Here's the drawing with two shaded views (mm, measured from the low corner). I have some questions. Round coordinates to 2 decimals unless told otherwise and drop trailing zeros. Order: outer loops, then holes, each group sorted by start corner. A loop starts at its lowest first (then second) coordinate and runs counter-clockwise, first axis right, second up. Notation, with made-up numbers: (-22, -35.5) -> (1, -35.5) arc R7 cw to (1, -22.5) -> close; hole circle Ø1 at (-24.5, 45). An arc over 180 degrees is marked (long way). Answer in a Markdown table with one row per item.
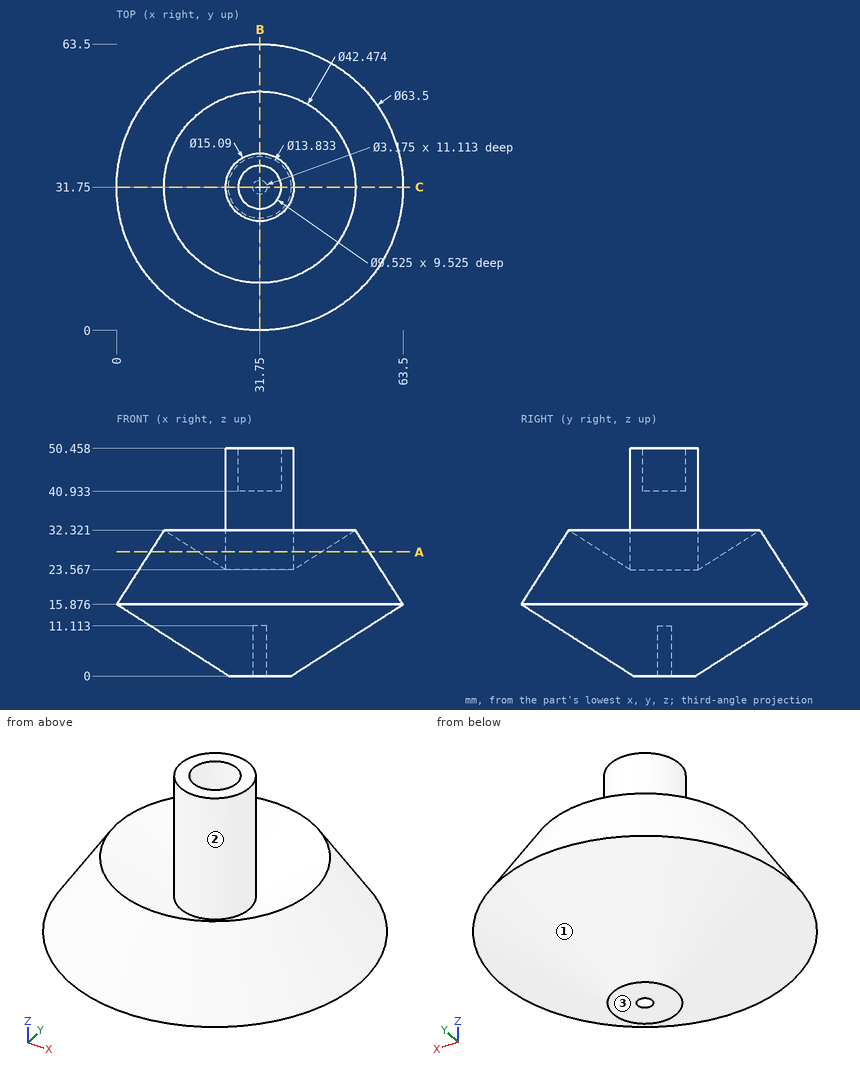
1. We'd pull the mould along X, two halves only. Please class the marked faces 1, 2 and 3: released by +X, released by -X, zero draft, split by the parting line, or undercut.
Numbers:
| item | result |
|---|---|
| face 1 | split by the parting line |
| face 2 | undercut |
| face 3 | zero draft |
2. Suppose I cut it at A-A on z = 27.5. State how many separate pieces and enclosed holes the cut face has, then the cut area to 3 significant figures.
Numbers:
| item | result |
|---|---|
| separate pieces | 2 |
| enclosed holes | 1 |
| area | 1,450 mm2 |
3. For pin 1 Ø10 at (x, y) = (10, 45) entering from +Z; pin 2 Ø1 at (x, y) = (47.5, 50.5) entering from +Z; pin 3 Ø6 at (x, y) = (38.5, 47) entering from -Z, each with a flat end and sliding along its axis, tell me the tip position at first contact or that it passes through.
Numbers:
| item | result |
|---|---|
| pin 1 | stops at z = 32.32 |
| pin 2 | stops at z = 28.02 |
| pin 3 | stops at z = 4.32 |
4. Suppose I cut it at B-B on x = 31.75. Write out the boundary of the cut face in (y, z) (1 decimal).
Numbers:
| item | result |
|---|---|
| outline | (0, 15.9) -> (24.8, 0) -> (30.2, 0) -> (30.2, 11.1) -> (33.3, 11.1) -> (33.3, 0) -> (38.7, 0) -> (63.5, 15.9) -> (53, 32.3) -> (39.3, 23.6) -> (39.3, 50.5) -> (36.5, 50.5) -> (36.5, 40.9) -> (27, 40.9) -> (27, 50.5) -> (24.2, 50.5) -> (24.2, 23.6) -> (10.5, 32.3) -> close |
5. Please list where these lines run through material, in increasing order: line 1 along Y through (x, z) = (31.75, 45) (1 decimal); line 2 along Y through (x, z) = (32, 7.5) (1 decimal); line 3 along X through (y, z) = (31, 45).
Numbers:
| item | result |
|---|---|
| line 1 | y = 24.2 to 27, 36.5 to 39.3 |
| line 2 | y = 13.1 to 30.2, 33.3 to 50.4 |
| line 3 | x = 24.24 to 27.05, 36.45 to 39.26 |
